Read the model definition and answer for the solid it produces. Units are mm, in the model's axes. A direction names the side the tool comes from. Give positions to 0.01 mm unless a question says otherwise; leave off trailing zeros. Order: outer loops, then holes, each group sorted by start corner. A loop starts at its lowest first (then second) coordinate and runs counter-clockwise, first axis right, second up.
Item 1: Given pin 1 Ø4 at (x, y) = (84.5, 49.5) entering from -Z; pin 2 Ø1.5 at (x, z) = (26.5, 85) entering from +Y; pin 3 Ø1.5 at (x, y) = (109.5, -155.5) entering from -Z, each flat-ended and moving along its own axis, determine where each tip first touches the part or whether it passes through.
Item 2: A cutting plane is placed at B-B (z = -76.5). Write down the section's boundary in (x, y), plus the area to 3 significant figures.
Item 3: Which of the six approach directions +Z, -Z, +X, -X, +Y, -Y give full straight-line access (tool end or side, diameter ignored) to faces 4 (the face through (83.11, 0.73, 39.98)), 5 (the face through (0, -29, 36))?
Item 4: The mould has two halves that part along Z. Classify faces 1 (the face through (83.109, 4.164, 78.747)), 2 (the face through (83.109, -187.326, 114.006)), 3 (the face through (83.109, -38.224, -59.742)): +Z half, -Z half, draft (parallel to the pull), parting line (faces both ways), or undercut.
Item 5: Find the intervals of material crossed by line 1 along Y through (x, z) = (97, 52.5); line 2 along Z through (x, y) = (47, 94); line 3 along Z through (x, y) = (128, 89), in increasing order.
Item 6: A cutting plane is placed at C-C (y = -135). Write down the section's boundary in (x, z).
Item 7: A cutting plane is placed at A-A (x = 42). Write down the section's boundary in (y, z).
from build123d import *

# Parameters (mm, degrees)
F0_R     = 27.2385686344
F1_DEPTH = 168.578363955
F2_DEPTH = 106.8018544465


with BuildPart() as f1:
    # F0 (on Right) → F1 (new body)
    with BuildSketch(Plane.YZ):
        Polygon((42.5867140293, 80.6694477797), (-13.1449922919, 13.4008079767), (-200.8079886436, 63.1083771586), (-160.7436537743, -22.5856415927), (87.7742916346, -97.9538932443), (147.1385359764, -4.5265853405), align=None)
        with Locations((62.3324811459, 0)):
            Circle(F0_R, mode=Mode.SUBTRACT)
    extrude(amount=F1_DEPTH)

    # F2 (add): faces of the model
    f2_faces = [f1.faces().sort_by_distance(p)[0] for p in [
        (84.2891819775, -106.9764904678, 38.2545925677),
        (84.2891819775, -36.4846810699, -60.2697674185),
    ]]
    extrude(f2_faces, amount=F2_DEPTH, dir=(0, 0.2560469353, 0.9666643507))


solid = f1.part
Response values:
1. pin 1: stops at z = -86.95
1. pin 2: stops at y = 6.02
1. pin 3: stops at z = -24.4
2. outline: (0, 17.03) - (168.58, 17.03) - (168.58, 101.41) - (0, 101.41) - close
2. area: 14,200 mm2
3. face 4: +X, -X
3. face 5: +Z, -Z, -X, +Y, -Y
4. face 1: undercut
4. face 2: +Z half
4. face 3: -Z half
5. line 1: y = -195.85 to -2.79, 19.25 to 77.16
5. line 2: z = -88.16 to 38.77
5. line 3: z = -96.02 to 42.85
6. outline: (0, -30.39) - (168.58, -30.39) - (168.58, 156.16) - (0, 156.16) - close
7. outline: (-200.81, 63.11) - (-160.74, -22.59) - (87.77, -97.95) - (147.14, -4.53) - (42.59, 80.67) - (7.24, 38) - (-5.6, 41.9) - (14.2, 116.64) - (-173.46, 166.35) - close; hole (50.95, 24.75) - (85.54, 14.26) arc R27.24 ccw to start
